Geometry: see drawing. Coordinates: mm, zero at the bounding-box minimum. A direction names the side the tool comes from. Give positions to 0.01 mm unless a question says otherwise; leave off trailing zeros. Loops run counter-clockwise (first coordinate to the right, second up) from the corner with the lowest first, then second, coordinate; pieces in that order, holes last. Notation, with made-up numbers: (9, 76.5) -> (64, 76.5) arc R6 cw to (64, 81.5) -> close; hole circle Ø3 at (-12.5, 80). An arc over 180 degrees is marked (long way). Return JSON: item names as keys, results as strings. Group by question number.
(1) Ray query, line 1 (Z direction, x = 7.5, y = 5); line 2 (X direction, y = 5.75, z = 22); line 3 (X direction, y = 2.5, z = 3.5). Return the intervals inside material, ascending. Write a range as from..to.
(2) Pin query (flat end, axial travel): pin 1 (2 mm diameter, centred on y = 9.5, z = 25, fed in from +X); pin 2 (1.5 mm diameter, centred on y = 5, z = 7.5, fed in from -X); pin 3 (1.5 mm diameter, centred on x = 7, z = 8.5, fed in from +Y); pin 4 (5 mm diameter, centred on y = 1.5, z = 29, fed in from -X). Return the tip coordinate at first contact, or that it passes through.
(3) Cut plane A-A on z = 35. Return loops of the section in (x, y).
(4) Cut plane B-B on z = 19. Return loops of the section in (x, y).
(5) Access query for the marked faces 1, 2 and 3. Directions: +Z, -Z, +X, -X, +Y, -Y. A direction counts if a zero-diameter tool reaches every point of the face in a straight line with its end or side. Return the directions, or none.
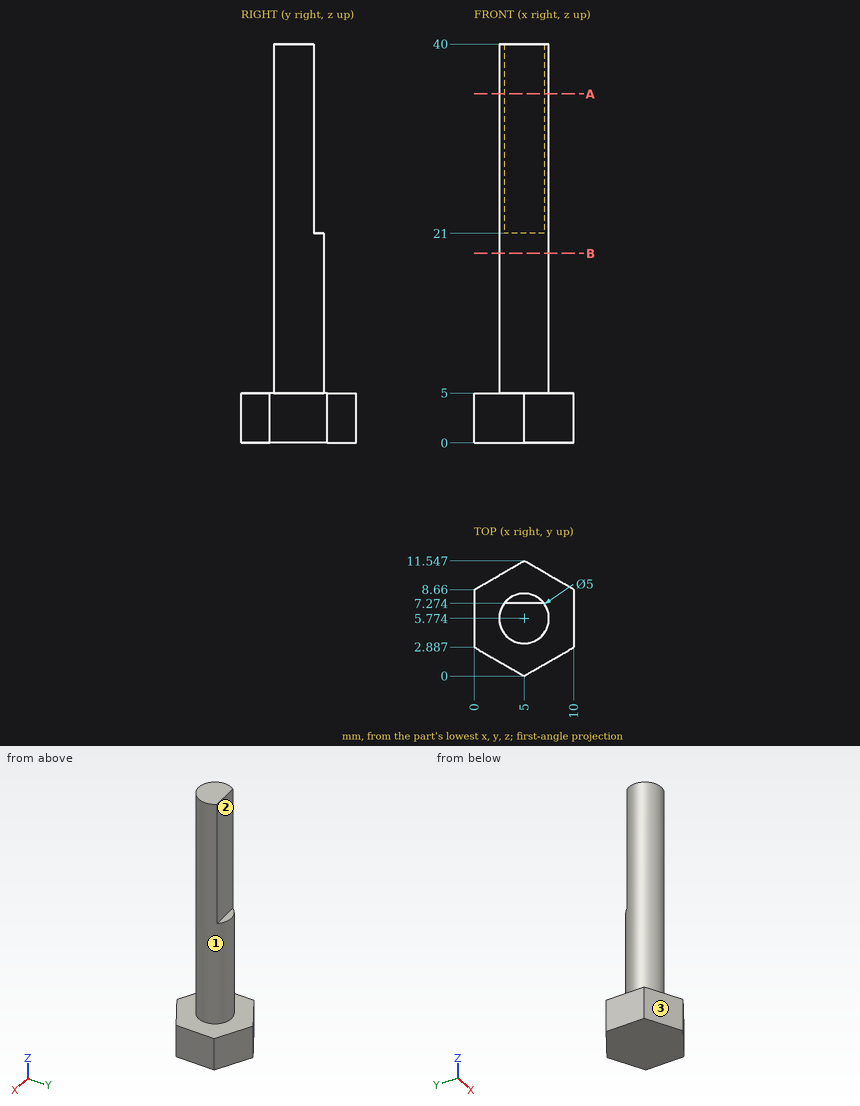
Answers:
{
 "1": {"line 1": "0..5", "line 2": "2.5..7.5", "line 3": "0.67..9.33"},
 "2": {"pin 1": "through", "pin 2": "x = 2.5", "pin 3": "y = 7.94", "pin 4": "x = 3.24"},
 "3": {"outline": "(3, 7.27) arc R2.5 ccw (long way) to (7, 7.27) -> close"},
 "4": {"outline": "circle Ø5 at (5, 5.77)"},
 "5": {"face 1": "+Z", "face 2": "+Z, +X, -X, +Y", "face 3": "+Z, -Z, -X, -Y"}
}
